Geometry check sheet. Reference: the model listing, model coordinates, mm. A direction names the side the tool comes from. Coordinates: 2 decimals unless noted, no trailing zeros. Write each loop counter-clockwise with the first axis right and the second up, starting at its lowest first coordinate (ties: lowest second). Pieces come first, ordered by that corner, then holes. Notation, with made-up numbers: (55, 26) - (107, 26) arc R21 ccw to (107, 49) - close; hole circle Ø7 at (13, -22). An arc over 180 degrees is marked (long way). Answer as a JSON object with one key per item and string values. Group by question number.
Autodesk Inventor part; units mm, degrees
ref_plane "YZ Plane" through (0, 0, 0) normal (1, 0, 0) x (0, 1, 0)
ref_plane "XZ Plane" through (0, 0, 0) normal (0, 1, 0) x (-1, 0, 0)
ref_plane "XY Plane" through (0, 0, 0) normal (0, 0, 1) x (1, 0, 0)
sketch "スケッチ1" plane through (0, 0, 0) normal (0, 0, 1) x (1, 0, 0)
  circle A0 centre (14.5, 10.5) radius 1.25
  circle A1 centre (14.5, -10.5) radius 1.25
  circle A2 centre (2, -10.5) radius 1.25
  circle A3 centre (2, 10.5) radius 1.25
  circle A4 centre (2.5, 0) radius 7
  line L0 (16.5, 12.5) -> (16.5, -12.5)
  line L1 (16.5, -12.5) -> (-7, -12.5)
  line L2 (-7, -12.5) -> (-7, 12.5)
  line L3 (-7, 12.5) -> (16.5, 12.5)
  circle A5 centre (2.5, 0) radius 7
  circle A6 centre (2, -10.5) radius 2.5
  circle A7 centre (2, 10.5) radius 2.5
  circle A8 centre (14.5, 10.5) radius 2.5
  circle A9 centre (14.5, -10.5) radius 2.5
  point P0 (0, 0)
  dimension "d0" = 2.5
  dimension "d1" = 2.5
  dimension "d2" = 2.5
  dimension "d3" = 2.5
  dimension "d4" = 2
  dimension "d5" = 2
  dimension "d6" = 2
  dimension "d7" = 9
extrude "押し出し1" add sketch "スケッチ1" along normal blind 1 contours A4 | L0 A8 L3 | L0 A8 L3 | L0 A9 L1 A6 L2 L3 A7 A8 | L0 A9 L1 | A7 L3 | L0 L1 A9 | L1 A6 picked at (2.0502, 12.247) picked at (2.0502, -12.247)
sketch "スケッチ2" plane through (0, 0, 0) normal (0, 0, -1) x (-1, 0, 0)
  circle A0 centre (-2, 10.5) radius 1.25
  circle A1 centre (-14.5, -10.5) radius 1.25
  circle A2 centre (-2, -10.5) radius 1.25
  circle A3 centre (-14.5, 10.5) radius 1.25
  circle A4 centre (-2.5, 0) radius 7
  line L0 (17.5, -15.5) -> (-17.5, -15.5)
  line L1 (-17.5, 15.5) -> (-17.5, -15.5)
  line L2 (-17.5, 15.5) -> (17.5, 15.5)
  line L3 (17.5, -15.5) -> (17.5, 15.5)
  line L4 (-6.5, 4) -> (1.5, 4)
  line L5 (1.5, 4) -> (1.5, -4)
  line L6 (1.5, -4) -> (-6.5, -4)
  line L7 (-6.5, -4) -> (-6.5, 4)
  line L8 (-6.5, 4) -> (1.5, -4) construction
  line L9 (1.5, 4) -> (-6.5, -4) construction
  point P0 (0, 0)
  dimension "d10" = 8
  dimension "d11" = 8
extrude "押し出し2" add sketch "スケッチ2" along normal blind 4 contours L4 L5 L6 L7
sketch "スケッチ3" plane through (0, 0, -4) normal (0, 0, -1) x (-1, 0, 0)
  circle A0 centre (-2.5, 0) radius 7
  circle A1 centre (-2.5, 0) radius 3.75
  point P0 (0, 0)
  dimension "d14" = 7.5
extrude "押し出し3" add sketch "スケッチ3" along normal blind 1 contours A1
properties part number "camerapi"
(1) Set-up check for faces 1 (the face through (3, 4, -2)), 2 (the face through (2, -4, -2)), 3 (the face through (-1.5, 0, -2)), 4 (the face through (6.246, -0.165, -4.493)): record each of +Z, -Z, +X, -X, +Y, -Y from which the full face is reachable in a straight line by a thin tool's end or side.
(2) Section check B-B (y = -10.5). Record the cut outline in (x, z), and give its area (3 significant figures).
(3) Section check D-D (y = 0). Record the cut outline in (x, z).
(4) Draft check along X on faces 5 (the face through (5, 0, 1)), 6 (the face through (6.5, 0, -2)), 7 (the face through (2.672, 9.446, 0.493)). Enter one of: +X half, -X half, draft (parallel to the pull), parting line (faces both ways), or undercut.
(5) Gauge pin test, flat ends, axial feed: pin 1 (1.5 mm diameter, centred on y = 1.5, z = -2.5, fed in from -X); pin 2 (6 mm diameter, centred on x = 1, y = -9.5, fed in from -Z); pin 3 (1.2 mm diameter, centred on x = 2, z = -1.5, fed in from +Y). Record the tip position at first contact, or that the pin passes through.
(6) Section check C-C (x = 2.5). Record the cut outline in (y, z), and give its area (3 significant figures).
(7) Material ranges on L1, parallel to Y at x = 2, z = 0.85; L2, parallel to Z at x = -3.25, y = 0; L3, parallel to X at y = -1, z = -2.5, recorded low to high. Write a range as [from, to].
(8) Section check A-A (z = 0.5). Record the cut outline in (x, y).
Conclusion:
{
 "1": {"face 1": "-Z, +X, -X, +Y", "face 2": "-Z, +X, -X, -Y", "face 3": "-Z, -X, +Y, -Y", "face 4": "-Z"},
 "2": {"outline": "(-7, 0) - (0.75, 0) - (0.75, 1) - (-7, 1) - close; (3.25, 0) - (13.25, 0) - (13.25, 1) - (3.25, 1) - close; (15.75, 0) - (16.5, 0) - (16.5, 1) - (15.75, 1) - close", "area": "18.5 mm^2"},
 "3": {"outline": "(-7, 0) - (-1.5, 0) - (-1.5, -4) - (-1.25, -4) - (-1.25, -5) - (6.25, -5) - (6.25, -4) - (6.5, -4) - (6.5, 0) - (16.5, 0) - (16.5, 1) - (-7, 1) - close"},
 "4": {"face 5": "draft", "face 6": "+X half", "face 7": "undercut"},
 "5": {"pin 1": "stops at x = -1.5", "pin 2": "stops at z = 0", "pin 3": "stops at y = 4"},
 "6": {"outline": "(-12.5, 0) - (-11.65, 0) - (-11.65, 1) - (-12.5, 1) - close; (-9.35, 0) - (-4, 0) - (-4, -4) - (-3.75, -4) - (-3.75, -5) - (3.75, -5) - (3.75, -4) - (4, -4) - (4, 0) - (9.35, 0) - (9.35, 1) - (-9.35, 1) - close; (11.65, 0) - (12.5, 0) - (12.5, 1) - (11.65, 1) - close", "area": "59.9 mm^2"},
 "7": {"L1": "y = [-12.5, -11.75], [-9.25, 9.25], [11.75, 12.5]", "L2": "z = [0, 1]", "L3": "x = [-1.5, 6.5]"},
 "8": {"outline": "(-7, -12.5) - (16.5, -12.5) - (16.5, 12.5) - (-7, 12.5) - close; hole circle Ø2.5 at (2, -10.5); hole circle Ø2.5 at (2, 10.5); hole circle Ø2.5 at (14.5, -10.5); hole circle Ø2.5 at (14.5, 10.5)"}
}
